Autodesk Inventor part; units mm, degrees
ref_plane "YZ Plane" through (0, 0, 0) normal (1, 0, 0) x (0, 1, 0)
ref_plane "XZ Plane" through (0, 0, 0) normal (0, 1, 0) x (-1, 0, 0)
ref_plane "XY Plane" through (0, 0, 0) normal (0, 0, 1) x (1, 0, 0)
sketch "Sketch1" plane through (0, 0, 0) normal (0, 1, 0) x (-1, 0, 0)
  line L0 (-85, 85) -> (85, 85)
  line L1 (85, 85) -> (85, -85)
  line L2 (85, -85) -> (-85, -85)
  line L3 (-85, -85) -> (-85, 85)
  line L4 (-85, 85) -> (85, -85) construction
  line L5 (85, 85) -> (-85, -85) construction
  point P0 (0, 0)
  dimension "d0" = 170
  dimension "d1" = 170
extrude "Extrusion1" add sketch "Sketch1" along normal blind 70
fillet "Fillet1" radius 5 8 edges at (0, 70, 85) (85, 70, 0) (-85, 70, 0) (-85, 35, 85) (85, 35, 85) (85, 35, -85) (0, 70, -85) (-85, 35, -85)
shell "Shell1" thickness 4 removed faces 1 at (28.3333, 0, -26.6667)
sketch "Sketch2" plane through (85, 0, 80) normal (1, 0, 0) x (0, 0, -1)
  point P0 (80, 0)
  point P1 (32.5535, 30.9629)
hole "Hole1" at (85, 30.9629, 47.4465) direction (-1, 0, 0) diameter 5 depth 8 tip angle 118
sketch "Sketch3" plane through (-80, 0, 85) normal (0, 0, 1) x (1, 0, 0)
  point P0 (80, 0)
  point P1 (124.013, 31.3444)
hole "Hole2" at (44.013, 31.3444, 85) direction (0, 0, -1) diameter 5 depth 8 tip angle 118
sketch "Sketch4" plane through (-85, 0, -80) normal (-1, 0, 0) x (0, 0, 1)
  point P0 (80, 0)
  point P1 (111.1547, 31.0118)
hole "Hole3" at (-85, 31.0118, 31.1547) direction (1, 0, 0) diameter 5 depth 8 tip angle 118
sketch "Sketch5" plane through (0, 70, 0) normal (0, 1, 0) x (1, 0, 0)
  circle A0 centre (-55.5639, 68.1591) radius 2.5
  circle A1 centre (-49.0639, 68.1591) radius 2.5
  point P0 (0, 0)
  dimension "d27" = 5
  dimension "d28" = 5
  dimension "d29" = 6.5
extrude "Extrusion2" cut sketch "Sketch5" against normal through all
properties part number "PCB_Housing_02"
The listing builds one solid part. Answer for the finished solid, in the listing's coordinates (mm). A direction names the side the tool comes from. Coordinates: 2 decimals unless noted, no trailing zeros. Loops run counter-clockwise (first coordinate to the right, second up) from the corner with the lowest first, then second, coordinate; pieces in that order, holes last. Notation, with made-up numbers: (-18.75, 41) -> (1.25, 41) arc R23 ccw to (1.25, 77) -> close; hole circle Ø1 at (20, 51.5). An arc over 180 degrees is marked (long way). Return JSON: item names as keys, results as strings. Group by question number.
(1) Given pin 1 Ø6.5 at (y, z) = (31.01, 31.15) entering from -X; pin 2 Ø8 at (x, z) = (57.5, 8.5) entering from -Y, each flat-ended and moving along its own axis, determine where each tip first touches the part or whether it passes through.
(2) Find the intervals of material crossed by probe 1 along X at (y, z) = (32, -59); probe 2 along X at (y, z) = (33, 32.5), in increasing order. Write a range as from..to.
(3) Which of the six approach directions +Z, -Z, +X, -X, +Y, -Y give full straight-line access (tool end or side, diameter ignored) to faces 5 (the flat face through (1, 32, 81)), 6 (the cylindrical face through (-83, 33, -84))?
(4) Determine the mould class of faces 1 (the cylindrical face through (42.323, 33.187, 82.972)), 2 (the cylindrical face through (82.972, 31.92, 45.137)), 3 (the cylindrical face through (-51.05, 68.03, -66.64)), 4 (the flat face through (1, 70, 1)) for opening direction Y: released by +Y, released by -Y, zero draft, split by the parting line, or undercut.
(5) A cutting plane is placed at C-C on x = 18. Write down the section's boundary in (y, z), and give its area (3 significant figures).
(6) A cutting plane is placed at B-B on z = 15.5. Write down the section's boundary in (x, y).
(7) A cutting plane is placed at A-A on y = 60.5. Write down the section's boundary in (x, z), and give its area (3 significant figures).
The answers:
{
 "1": {"pin 1": "stops at x = -85", "pin 2": "stops at y = 66"},
 "2": {"probe 1": "x = -85..-81, 81..85", "probe 2": "x = 81..85"},
 "3": {"face 5": "-Y", "face 6": "-Z, -X, +Y, -Y"},
 "4": {"face 1": "undercut", "face 2": "undercut", "face 3": "zero draft", "face 4": "released by +Y"},
 "5": {"outline": "(0, -85) -> (65, -85) arc R5 ccw to (70, -80) -> (70, 80) arc R5 ccw to (65, 85) -> (0, 85) -> (0, 81) -> (65, 81) arc R1 cw to (66, 80) -> (66, -80) arc R1 cw to (65, -81) -> (0, -81) -> close", "area": "1,200 mm^2"},
 "6": {"outline": "(-85, 0) -> (-81, 0) -> (-81, 65) arc R1 cw to (-80, 66) -> (80, 66) arc R1 cw to (81, 65) -> (81, 0) -> (85, 0) -> (85, 65) arc R5 ccw to (80, 70) -> (-80, 70) arc R5 ccw to (-85, 65) -> close"},
 "7": {"outline": "(-85, -80) arc R5 ccw to (-80, -85) -> (80, -85) arc R5 ccw to (85, -80) -> (85, 80) arc R5 ccw to (80, 85) -> (-80, 85) arc R5 ccw to (-85, 80) -> close; hole (-81, -80) arc R1 ccw to (-80, -81) -> (80, -81) arc R1 ccw to (81, -80) -> (81, 80) arc R1 ccw to (80, 81) -> (-80, 81) arc R1 ccw to (-81, 80) -> close", "area": "2,640 mm^2"}
}
